Input: part model. Units: mm. Frame: model coordinates. Face numbers are marked on the shaded views. A direction names the side the tool comes from. Coordinates: 2 decimals unless noted, no trailing zeros. Write each loop counter-clockwise with the first axis right and the second up, starting at its lowest first coordinate (ties: lowest second). Pieces come first, ordered by that corner, then holes. Notation, with made-up numbers: (-39.5, -1.75) - (-0.5, -1.75) arc R16 ccw to (-0.5, 9.25) - close; hole circle Ø8 at (53, 28.25). An arc over 180 degrees is marked (long way). Use a Markdown table: item, result. Add a question column.
Q1. Section query B-B (y = 0). Return the cut outline in (x, z).
Q2. Section query D-D (y = -2). Return the cut outline in (x, z), then the cut area to 3 significant figures.
Q3. Pin query (flat end, axial travel): P1, Ø12, axis at y = 7.5, z = 10.5, coming from the +X side; P2, Ø10, axis at x = -7, z = 6, coming from the +Y side; P3, Ø1, axis at x = -10.5, z = 8, coming from the -Y side. Return the tip coordinate at first contact, or that it passes through.
Q4. Section query A-A (x = 10). Return the cut outline in (y, z).
Q5. Set-up query: the marked faces 1 and 2. Return all of +Z, -Z, +X, -X, +Y, -Y with unobstructed straight access to the full face (end or side cutting, diameter ignored); none if empty.
Q6. Section query C-C (z = 20.5). Return the cut outline in (x, y), then the cut area to 3 significant figures.
Q7. Mould query, pull axis X, two halves, no side actions, for the marked faces 3, 4, 5 and 6. Classes: released by +X, released by -X, zero draft, split by the parting line, or undercut.
Q8. Material intervals for probe 1 along Y at (x, z) = (10, 2.25); probe 2 along Z at (x, y) = (16, -2.5); probe 3 along X at (y, z) = (0.5, 8), sorted ascending. Write a range as from..to.
from build123d import *

# Parameters (mm, degrees)
F0_W     = 40
F0_H     = 20
F0_R     = 4
F1_DEPTH = 3
F2_R     = 4
F3_DEPTH = 25
F4_R     = 5


with BuildPart() as f1:
    # F0 (on Top) → F1 (new body)
    with BuildSketch(Plane.XY):
        Rectangle(F0_W, F0_H)
        with Locations((-10, 0)):
            Circle(F0_R, mode=Mode.SUBTRACT)
        with Locations((10, 0)):
            Circle(F0_R, mode=Mode.SUBTRACT)
        with Locations((-10, 0)):
            Circle(F0_R)
        with Locations((10, 0)):
            Circle(F0_R)
    extrude(amount=-F1_DEPTH)

    # F2 (on face) → F3 (join)
    with BuildSketch(Plane.XY):
        with Locations((-10, 0)):
            Circle(F2_R)
        with Locations((10, 0)):
            Circle(F2_R)
    extrude(amount=F3_DEPTH)

    # F4
    f4_edges = [f1.edges().sort_by_distance(p)[0] for p in [
        (-20, -10, -1.5),
        (-20, 10, -1.5),
        (20, 10, -1.5),
        (20, -10, -1.5),
    ]]
    fillet(f4_edges, radius=F4_R)


solid = f1.part
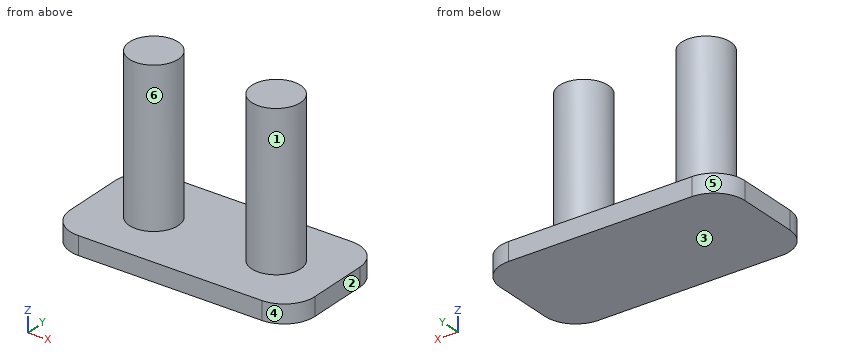
Values follow:
| question | item | result |
|---|---|---|
| 1 | outline | (-20, -3) - (20, -3) - (20, 0) - (14, 0) - (14, 25) - (6, 25) - (6, 0) - (-6, 0) - (-6, 25) - (-14, 25) - (-14, 0) - (-20, 0) - close |
| 2 | outline | (-20, -3) - (20, -3) - (20, 0) - (13.46, 0) - (13.46, 25) - (6.54, 25) - (6.54, 0) - (-6.54, 0) - (-6.54, 25) - (-13.46, 25) - (-13.46, 0) - (-20, 0) - close |
| 2 | area | 466 mm2 |
| 3 | P1 | x = 13.71 |
| 3 | P2 | y = 4 |
| 3 | P3 | y = -4 |
| 4 | outline | (-10, -3) - (10, -3) - (10, 0) - (4, 0) - (4, 25) - (-4, 25) - (-4, 0) - (-10, 0) - close |
| 5 | face 1 | +Z |
| 5 | face 2 | +Z, -Z, +X, +Y, -Y |
| 6 | outline | circle Ø8 at (-10, 0); circle Ø8 at (10, 0) |
| 6 | area | 101 mm2 |
| 7 | face 3 | zero draft |
| 7 | face 4 | released by +X |
| 7 | face 5 | released by -X |
| 7 | face 6 | undercut |
| 8 | probe 1 | -4..4 |
| 8 | probe 2 | -3..0 |
| 8 | probe 3 | -13.97..-6.03, 6.03..13.97 |
